CAD build for the part. Positions are in the model's coordinates, mm. Round coordinates to 2 decimals unless told otherwise and drop trailing zeros. Write each loop counter-clockwise with the first axis right and the second up, starting at its lowest first coordinate (ties: lowest second). Pieces come first, ordered by that corner, then holes. Notation, with made-up numbers: (41, 24.5) - (72, 24.5) arc R20 cw to (72, 44.5) - close; hole circle Ø11 at (6.25, 82.5). An arc over 180 degrees is marked (long way). Put each result on its own line as item: value. Start each with the question number.
Item 1: Pin check, flat tips, straight feed: pin 1 Ø1.6 at (y, z) = (2, 3.5) entering from -X; pin 2 Ø2.5 at (y, z) = (99, 3.5) entering from +X; pin 3 Ø1 at (x, z) = (19.5, 2) entering from +Y. Stop position of each tip, or through.
Item 2: Cut at A-A (y = 109). Give the cut face in (x, z).
Item 3: Cut at C-C (x = 5). Count the separate pieces of the cut face and the enclosed holes in it, and give its area (3 significant figures).
Item 4: Cut at B-B (y = 39). Give the cut face in (x, z), and give its area (3 significant figures).
Item 5: Drill centre lines: line 1 (X direction, y = 83, z = 3.1); line 2 (X direction, y = 92.5, z = 2.2); line 3 (X direction, y = 75, z = 1.15). Where is each one in solid material? Low to high. Write a range as from..to.
```python
from build123d import *

# Parameters (mm, degrees)
EXTRUDE_1_DEPTH     = 5
SKETCH_2_R          = 1.6
SKETCH_2_W          = 7.5
SKETCH_2_H          = 3.1
CUT_EXTRUDE_1_DEPTH = 5
EXTRUDE_START       = -2.5
SKETCH_3_R          = 2.6
EXTRUDE_2_DEPTH     = 2.5


with BuildPart() as part:
    # 草图1 → 凸台-拉伸1 (new body)
    with BuildSketch(Plane.XY):
        with BuildLine():
            Line((0, 0), (45, 0))
            Line((45, 0), (45, 113.1))
            ThreePointArc((45, 113.1), (22.5, 152.07114317), (0, 113.1))
            Line((0, 113.1), (0, 0))
        make_face()
        with BuildLine():
            Line((19.44, 129.02), (25.56, 129.02))
            ThreePointArc((25.56, 129.02), (22.5, 138.2), (19.44, 129.02))
        make_face(mode=Mode.SUBTRACT)
    extrude(amount=EXTRUDE_1_DEPTH)

    # 草图2 → 切除-拉伸1 (cut)
    with BuildSketch(Plane.XY.offset(5)):
        with Locations((40, 8.1)):
            Circle(SKETCH_2_R)
        with Locations((5, 8.1)):
            Circle(SKETCH_2_R)
        with Locations((31.25, 1.55)):
            Rectangle(SKETCH_2_W, SKETCH_2_H)
        with Locations((13.75, 1.55)):
            Rectangle(SKETCH_2_W, SKETCH_2_H)
        Polygon((7.5, 26), (2.303847577, 23), (2.303847577, 17), (7.5, 14), (12.696152423, 17), (12.696152423, 23), align=None)
        Polygon((22.5, 26), (17.303847577, 23), (17.303847577, 17), (22.5, 14), (27.696152423, 17), (27.696152423, 23), align=None)
        Polygon((37.5, 26), (32.303847577, 23), (32.303847577, 17), (37.5, 14), (42.696152423, 17), (42.696152423, 23), align=None)
        Polygon((15, 56), (9.803847577, 53), (9.803847577, 47), (15, 44), (20.196152423, 47), (20.196152423, 53), align=None)
        Polygon((15, 36), (9.803847577, 33), (9.803847577, 27), (15, 24), (20.196152423, 27), (20.196152423, 33), align=None)
        Polygon((30, 36), (24.803847577, 33), (24.803847577, 27), (30, 24), (35.196152423, 27), (35.196152423, 33), align=None)
        Polygon((30, 56), (24.803847577, 53), (24.803847577, 47), (30, 44), (35.196152423, 47), (35.196152423, 53), align=None)
        Polygon((37.5, 46), (32.303847577, 43), (32.303847577, 37), (37.5, 34), (42.696152423, 37), (42.696152423, 43), align=None)
        Polygon((22.5, 46), (17.303847577, 43), (17.303847577, 37), (22.5, 34), (27.696152423, 37), (27.696152423, 43), align=None)
        Polygon((7.5, 46), (2.303847577, 43), (2.303847577, 37), (7.5, 34), (12.696152423, 37), (12.696152423, 43), align=None)
        Polygon((15, 76), (9.803847577, 73), (9.803847577, 67), (15, 64), (20.196152423, 67), (20.196152423, 73), align=None)
        Polygon((30, 76), (24.803847577, 73), (24.803847577, 67), (30, 64), (35.196152423, 67), (35.196152423, 73), align=None)
        Polygon((37.5, 66), (32.303847577, 63), (32.303847577, 57), (37.5, 54), (42.696152423, 57), (42.696152423, 63), align=None)
        Polygon((22.5, 66), (17.303847577, 63), (17.303847577, 57), (22.5, 54), (27.696152423, 57), (27.696152423, 63), align=None)
        Polygon((7.5, 66), (2.303847577, 63), (2.303847577, 57), (7.5, 54), (12.696152423, 57), (12.696152423, 63), align=None)
        Polygon((15, 96), (9.803847577, 93), (9.803847577, 87), (15, 84), (20.196152423, 87), (20.196152423, 93), align=None)
        Polygon((30, 96), (24.803847577, 93), (24.803847577, 87), (30, 84), (35.196152423, 87), (35.196152423, 93), align=None)
        Polygon((37.5, 86), (32.303847577, 83), (32.303847577, 77), (37.5, 74), (42.696152423, 77), (42.696152423, 83), align=None)
        Polygon((22.5, 86), (17.303847577, 83), (17.303847577, 77), (22.5, 74), (27.696152423, 77), (27.696152423, 83), align=None)
        Polygon((7.5, 86), (2.303847577, 83), (2.303847577, 77), (7.5, 74), (12.696152423, 77), (12.696152423, 83), align=None)
        Polygon((15, 116), (9.803847577, 113), (9.803847577, 107), (15, 104), (20.196152423, 107), (20.196152423, 113), align=None)
        Polygon((30, 116), (24.803847577, 113), (24.803847577, 107), (30, 104), (35.196152423, 107), (35.196152423, 113), align=None)
        Polygon((37.5, 106), (32.303847577, 103), (32.303847577, 97), (37.5, 94), (42.696152423, 97), (42.696152423, 103), align=None)
        Polygon((22.5, 106), (17.303847577, 103), (17.303847577, 97), (22.5, 94), (27.696152423, 97), (27.696152423, 103), align=None)
        Polygon((7.5, 106), (2.303847577, 103), (2.303847577, 97), (7.5, 94), (12.696152423, 97), (12.696152423, 103), align=None)
        Polygon((7.5, 126), (2.303847577, 123), (2.303847577, 117), (7.5, 114), (12.696152423, 117), (12.696152423, 123), align=None)
        Polygon((22.5, 126), (17.303847577, 123), (17.303847577, 117), (22.5, 114), (27.696152423, 117), (27.696152423, 123), align=None)
        Polygon((37.5, 126), (32.303847577, 123), (32.303847577, 117), (37.5, 114), (42.696152423, 117), (42.696152423, 123), align=None)
    extrude(amount=-CUT_EXTRUDE_1_DEPTH, mode=Mode.SUBTRACT)

    # 草图3 → 凸台-拉伸2 (add)
    with BuildSketch(Plane.XY.offset(5).offset(EXTRUDE_START)):
        with BuildLine():
            Line((19.44, 129.02), (25.56, 129.02))
            ThreePointArc((25.56, 129.02), (22.5, 138.2), (19.44, 129.02))
        make_face()
        with Locations((22.5, 133.1)):
            Circle(SKETCH_3_R, mode=Mode.SUBTRACT)
    extrude(amount=EXTRUDE_2_DEPTH)


solid = part.part
```
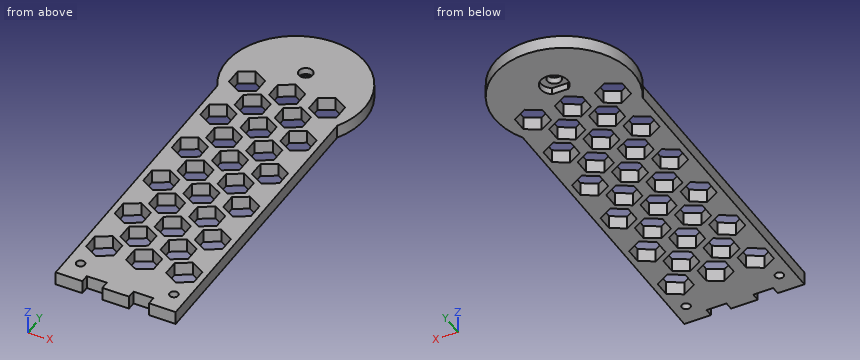
Output values:
1. pin 1: x = 0
1. pin 2: x = 45
1. pin 3: y = 151.95
2. outline: (0, 0) - (9.8, 0) - (9.8, 5) - (0, 5) - close; (20.2, 0) - (24.8, 0) - (24.8, 5) - (20.2, 5) - close; (35.2, 0) - (45, 0) - (45, 5) - (35.2, 5) - close
3. separate pieces: 8
3. enclosed holes: 0
3. area: 437 mm2
4. outline: (0, 0) - (2.3, 0) - (2.3, 5) - (0, 5) - close; (12.7, 0) - (17.3, 0) - (17.3, 5) - (12.7, 5) - close; (27.7, 0) - (32.3, 0) - (32.3, 5) - (27.7, 5) - close; (42.7, 0) - (45, 0) - (45, 5) - (42.7, 5) - close
4. area: 69.1 mm2
5. line 1: 0..2.3, 12.7..17.3, 27.7..32.3, 42.7..45
5. line 2: 0..9.8, 20.2..24.8, 35.2..45
5. line 3: 0..5.77, 9.23..13.27, 16.73..20.77, 24.23..28.27, 31.73..35.77, 39.23..45
